```python
from build123d import *

# Parameters (mm, degrees)
PAD_DEPTH    = 6.35
SKETCH001_R  = 3.175
PAD001_DEPTH = 25.4


with BuildPart() as part:
    # Sketch → Pad (new body)
    with BuildSketch(Plane.XY):
        Polygon((4.7625, 2.749631), (0, 5.499261), (-4.7625, 2.749631), (-4.7625, -2.749631), (0, -5.499261), (4.7625, -2.749631), align=None)
    extrude(amount=-PAD_DEPTH)

    # Sketch001 (on Face8 of Pad) → Pad001 (join)
    with BuildSketch(Plane(origin=(0, 0, -6.35), x_dir=(1, 0, 0), z_dir=(0, 0, -1))):
        Circle(SKETCH001_R)
    extrude(amount=PAD001_DEPTH)


solid = part.part
```
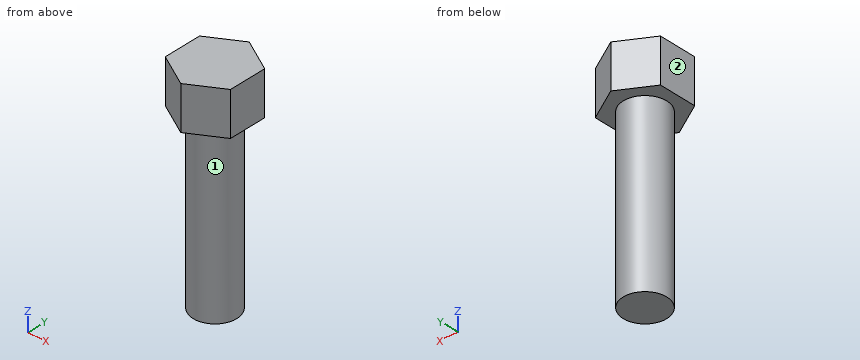
For this review, take the finished solid that the model builds, in its own axes (mm). Face numbers are marked on the shaded views. A direction names the side the tool comes from. Coordinates: 2 decimals unless noted, no trailing zeros. Loops run counter-clockwise (first coordinate to the right, second up) from the corner with the lowest first, then second, coordinate; pieces in that order, holes last. Notation, with made-up numbers: (9, 12) - (29, 12) arc R19 cw to (29, 31) - close; hole circle Ø11 at (71, 39.5). An arc over 180 degrees is marked (long way). Use one line per item in the form item = value. Start each with the question number.
1) Take a section at B-B (x = -1.5). State the section outline as (y, z) points, plus the area to 3 significant figures.
2) Take a section at C-C (y = 3.5). State the section outline as (x, z) points.
3) To check wall thickness, follow probe 1 along Z at (x, y) = (0.25, -3.75); probe 2 along X at (y, z) = (-3.75, -1); probe 3 along Y at (x, z) = (-0.75, -11). State the ranges of each line that lie inside material, in increasing order. Write a range as from..to.
4) For pin 1 (6 mm diameter, centred on y = -1.5, z = -24.5, fed in from +X) (3 decimals); pin 2 (6 mm diameter, centred on y = -2, z = -28, fed in from -X) (3 decimals); pin 3 (1.5 mm diameter, centred on y = -2.5, z = -21.5, fed in from -X), all flat-tipped, find the tip position at first contact; note any pin that passes through.
5) For the marked faces 1 and 2, list the 3-axis set-ups (+Z, -Z, +X, -X, +Y, -Y) from which the entire face can be reached by the end or side of a thin tool; tool diameter is ignored.
6) Take a section at D-D (x = 4.25). State the section outline as (y, z) points.
From the geometry:
q1.outline = (-4.63, -6.35) - (-2.8, -6.35) - (-2.8, -31.75) - (2.8, -31.75) - (2.8, -6.35) - (4.63, -6.35) - (4.63, 0) - (-4.63, 0) - close
q1.area = 201 mm2
q2.outline = (-3.46, -6.35) - (3.46, -6.35) - (3.46, 0) - (-3.46, 0) - close
q3.probe_1 = -6.35..0
q3.probe_2 = -3.03..3.03
q3.probe_3 = -3.09..3.09
q4.pin_1 = 3.175
q4.pin_2 = -3.175
q4.pin_3 = -2.65
q5.face_1 = -Z
q5.face_2 = +Z, -Z, -X, +Y, -Y
q6.outline = (-3.05, -6.35) - (3.05, -6.35) - (3.05, 0) - (-3.05, 0) - close
